The model under review builds one solid part; all positions refer to its coordinate system, in mm. A direction names the side the tool comes from. Round coordinates to 2 decimals unless told otherwise and drop trailing zeros. Order: outer loops, then holes, each group sorted by start corner. A loop starts at its lowest first (then second) coordinate and runs counter-clockwise, first axis right, second up. Notation, with made-up numbers: (-19.5, -11) -> (1.5, -11) arc R33 cw to (1.5, 23) -> close; hole circle Ø9 at (-33.5, -34.5). An arc over 180 degrees is marked (long way). Return JSON: item names as keys, results as strings. Group by question number.
from build123d import *

# Parameters (mm, degrees)
SKETCH2_R           = 25
BOSS_EXTRUDE1_DEPTH = 10
SKETCH3_R           = 20
BOSS_EXTRUDE2_DEPTH = 8
BOSS_EXTRUDE3_DEPTH = 20
SKETCH5_R           = 12.5
CUT_EXTRUDE1_DEPTH  = 52.903757089


with BuildPart() as part:
    # Sketch2 → Boss-Extrude1 (new body)
    with BuildSketch(Plane.XY):
        Circle(SKETCH2_R)
    extrude(amount=BOSS_EXTRUDE1_DEPTH)

    # Sketch3 → Boss-Extrude2 (add)
    with BuildSketch(Plane.XY.offset(10)):
        Circle(SKETCH3_R)
    extrude(amount=BOSS_EXTRUDE2_DEPTH)

    # Sketch4 → Boss-Extrude3 (add)
    with BuildSketch(Plane(origin=(0, 0, 0), x_dir=(-1, 0, 0), z_dir=(0, 0, -1))):
        Polygon((-20.437108974, -9.047000469), (-2.383622252, -22.222555786), (18.053486721, -13.175555316), (20.437108974, 9.047000469), (2.383622252, 22.222555786), (-18.053486721, 13.175555316), align=None)
    extrude(amount=BOSS_EXTRUDE3_DEPTH)

    # Sketch5 → Cut-Extrude1 (cut, through all)
    with BuildSketch(Plane(origin=(0, 0, -20), x_dir=(-1, 0, 0), z_dir=(0, 0, -1))):
        Circle(SKETCH5_R)
    extrude(amount=-CUT_EXTRUDE1_DEPTH, mode=Mode.SUBTRACT)


solid = part.part
Item 1: Wall thickness on line 1 along Y through (x, z) = (0.5, 5) (3 decimals); line 2 along Z through (x, y) = (15.5, 15.5); line 3 along Y through (x, z) = (7, -4): over which ranges is each line inside the solid? List them lowest first.
Item 2: Insertion check: pin 1 Ø2 at (x, z) = (11, -12) entering from +Y; pin 2 Ø6 at (y, z) = (-4.5, -3.5) entering from +X; pin 3 Ø10 at (y, z) = (13, -12.5) entering from -X. Each pin has a flat end and moves straight along its axis. Give the tip position at first contact, or say it passes through.
Item 3: The part is to be moulded in two halves that separate along X. For faces 1 (the face through (19.23, 2.22, -9.86)), 2 (the face through (13, -15, 0)), 3 (the face through (-11.923, 3.755, -1.266)), 4 (the face through (-19.23, -2.22, -9.86)), say which applies: +X half, -X half, draft (parallel to the pull), parting line (faces both ways), or undercut.
Item 4: Consider section A-A on x = -9.5. State the section outline as (y, z) points.
Item 5: Consider section C-C on z = -6. State the section outline as (x, y) points.
Item 6: For faces 5 (the face through (-4.336, -19.524, 13.944)), 6 (the face through (7.692, 17.762, -9.86)), 7 (the face through (-11.54, 15.54, -9.86)), 8 (the face through (11.54, -15.54, -9.86)), list the 3-axis set-ups (+Z, -Z, +X, -X, +Y, -Y) from which the entire face can be reached by the end or side of a thin tool; tool diameter is ignored.
Item 7: Consider section D-D on y = -18. State the section outline as (x, z) points.
Item 8: Consider section B-B on y = -2. State the section outline as (x, z) points, plus the area to 3 significant figures.
Values:
{
 "1": {"line 1": "-24.995 to -12.49, 12.49 to 24.995", "line 2": "0 to 10", "line 3": "-18.85 to -10.36, 10.36 to 18.07"},
 "2": {"pin 1": "y = 16.74", "pin 2": "x = 20.27", "pin 3": "x = -20.44"},
 "3": {"face 1": "+X half", "face 2": "draft", "face 3": "undercut", "face 4": "-X half"},
 "4": {"outline": "(-23.12, 0) -> (-16.96, 0) -> (-16.96, -20) -> (-8.12, -20) -> (-8.12, 18) -> (-17.6, 18) -> (-17.6, 10) -> (-23.12, 10) -> close; (8.12, -20) -> (17.03, -20) -> (17.03, 0) -> (23.12, 0) -> (23.12, 10) -> (17.6, 10) -> (17.6, 18) -> (8.12, 18) -> close"},
 "5": {"outline": "(-20.44, 9.05) -> (-18.05, -13.18) -> (2.38, -22.22) -> (20.44, -9.05) -> (18.05, 13.18) -> (-2.38, 22.22) -> close; hole circle Ø25 at (0, 0)"},
 "6": {"face 5": "+Z", "face 6": "-Z, +X, +Y", "face 7": "-Z, -X, +Y", "face 8": "-Z, +X, -Y"},
 "7": {"outline": "(-17.35, 0) -> (-7.16, 0) -> (-7.16, -20) -> (8.17, -20) -> (8.17, 0) -> (17.35, 0) -> (17.35, 10) -> (8.72, 10) -> (8.72, 18) -> (-8.72, 18) -> (-8.72, 10) -> (-17.35, 10) -> close"},
 "8": {"outline": "(-24.92, 0) -> (-19.25, 0) -> (-19.25, -20) -> (-12.34, -20) -> (-12.34, 18) -> (-19.9, 18) -> (-19.9, 10) -> (-24.92, 10) -> close; (12.34, -20) -> (19.68, -20) -> (19.68, 0) -> (24.92, 0) -> (24.92, 10) -> (19.9, 10) -> (19.9, 18) -> (12.34, 18) -> close", "area": "658 mm^2"}
}
